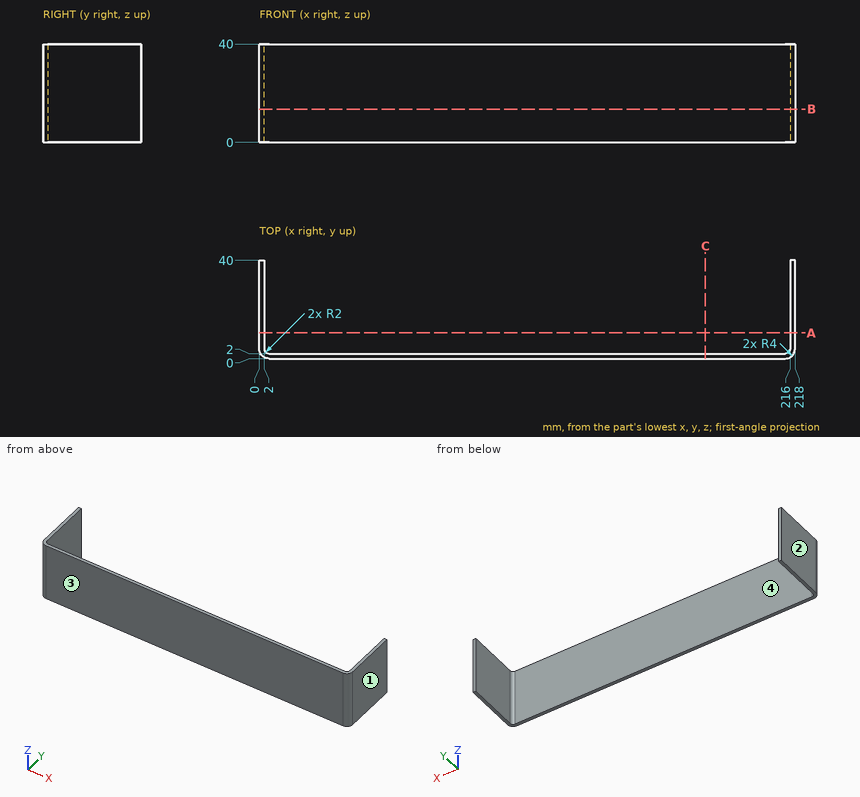
Here's the drawing with two shaded views (mm, measured from the low corner). I have some questions. Give positions to 0.01 mm unless a question says otherwise; leave off trailing zeros. Order: outer loops, then holes, each group sorted by start corner. A loop starts at its lowest first (then second) coordinate and runs counter-clockwise, first axis right, second up.
Q1. Suppose I cut it at A-A, the plane y = 10.5. Write out the boundary of the cut face in (x, z), and give its area (3 significant figures).
Q2. Suppose I cut it at B-B, the plane z = 13.5. Write out the boundary of the cut face in (x, y), and give its area (3 significant figures).
Q3. Suppose I cut it at C-C, the plane x = 181.5. Write out the boundary of the cut face in (y, z), and give its area (3 significant figures).
Q4. We'd pull the mould along X, two halves only. Please class the marked faces 1, 2, 3 and 4: +X half, -X half, draft (parallel to the pull), parting line (faces both ways), or undercut.
Q5. I'm going to push flat-ended pins straight in: P1, Ø1, axis at y = 12, z = 26, coming from the -X side; P2, Ø3, axis at x = 78, z = 20.5, coming from the +Y side. Where does each tip first touch, or does it pass through?
Q6. If I drill on line 1 along X through (y, z) = (20, 30.5); line 2 along Y through (x, z) = (78.5, 23); line 3 along X through (y, z) = (3, 33), over which ranges is the centre line in solid material (lowest first)?
Solution:
1. outline: (0, 0) - (2, 0) - (2, 40) - (0, 40) - close; (216, 0) - (218, 0) - (218, 40) - (216, 40) - close
1. area: 160 mm2
2. outline: (0, 4) arc R4 ccw to (4, 0) - (214, 0) arc R4 ccw to (218, 4) - (218, 40) - (216, 40) - (216, 4) arc R2 cw to (214, 2) - (4, 2) arc R2 cw to (2, 4) - (2, 40) - (0, 40) - close
2. area: 583 mm2
3. outline: (0, 0) - (2, 0) - (2, 40) - (0, 40) - close
3. area: 80.0 mm2
4. face 1: +X half
4. face 2: -X half
4. face 3: draft
4. face 4: undercut
5. P1: stops at x = 0
5. P2: stops at y = 2
6. line 1: x = 0 to 2, 216 to 218
6. line 2: y = 0 to 2
6. line 3: x = 0.13 to 2.27, 215.73 to 217.87
